For this review, take the finished solid that the model builds, in its own axes (mm). Face numbers are marked on the shaded views. A direction names the side the tool comes from. Give positions to 0.01 mm unless a question says otherwise; leave off trailing zeros. Order: outer loops, then holes, each group sorted by start corner. A loop starts at its lowest first (then second) coordinate and runs counter-clockwise, first axis right, second up. Notation, with made-up numbers: (29.5, 79) - (33.5, 79) arc R23 ccw to (33.5, 101) - close; hole circle Ø5 at (85, 13.5). An arc over 180 degrees is marked (long way). One line per item, written item: value.
Solid Edge part; units mm, degrees
sketch "Sketch1" plane through (0, 0, 0) normal (0, -1, 0) x (1, 0, 0)
  circle A0 centre (0, 0) radius 125
extrude "Protrusion1" add sketch "Sketch1" against normal blind 6
sketch "Sketch2" plane through (0, 0, 0) normal (0, -1, 0) x (1, 0, 0)
  circle A0 centre (0, 0) radius 25
extrude "ProtrusiónExtruida_2" add sketch "Sketch2" along normal blind 45
sketch "Sketch3" plane through (0, -45, 0) normal (0, -1, 0) x (1, 0, 0)
  line L0 (-5, 24.4949) -> (-5, 16.7705)
  line L1 (5, 24.4949) -> (5, 16.7705)
  arc A0 (5, 24.4949) -> (-5, 24.4949) centre (0, 0) cw
  arc A1 (5, 16.7705) -> (-5, 16.7705) centre (0, 0) cw
extrude "Cutout1" cut sketch "Sketch3" against normal up to surface (45 mm away)
sketch "Sketch4" plane through (0, 0, 0) normal (0, -1, 0) x (1, 0, 0)
  circle A0 centre (0, 0) radius 25
extrude "ProtrusiónExtruida_3" add sketch "Sketch4" along normal blind 15
fillet "Redondeo_1" radius 5 1 edges at (-25, 0, 0)
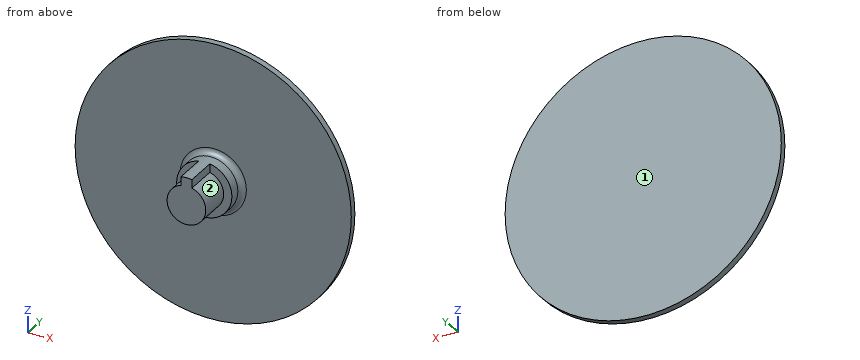
(1) Wall thickness on line 1 (X direction, y = -32, z = -0.5); line 2 (Y direction, x = 111.5, z = 41); line 3 (X direction, y = -10.5, z = 21.5): over which ranges is each line inside the solid? List them lowest first. Write a range as from..to.
Answers below:
line 1: x = -17.49..17.49
line 2: y = 0..6
line 3: x = -12.76..12.76
(2) Take a section at C-C (y = -38). Write out the cut boundary in (x, z).
Answers below:
outline: (-5, 16.77) arc R17.5 ccw (long way) to (5, 16.77) - (5, 24.49) arc R25 ccw to (-5, 24.49) - close
(3) Take a section at D-D (z = -74). Write out the cut boundary in (x, y), then the cut area to 3 significant figures.
Answers below:
outline: (-100.74, 0) - (100.74, 0) - (100.74, 6) - (-100.74, 6) - close
area: 1,210 mm^2
(4) For P1, Ø4, axis at y = -34.5, z = 19.5, coming from the -X side; P2, Ø6, axis at y = -27, z = 20.5, coming from the +X side; P3, Ø12, axis at x = 9.5, y = -17, coming from the -Z side, all flat-tipped, find the tip position at first contact; note any pin that passes through.
Answers below:
P1: stops at x = -5
P2: stops at x = 5
P3: stops at z = -24.7
(5) Take a section at B-B (z = 0). Write out the cut boundary in (x, y).
Answers below:
outline: (-125, 0) - (-30, 0) arc R5 cw to (-25, -5) - (-25, -15) - (-17.5, -15) - (-17.5, -45) - (17.5, -45) - (17.5, -15) - (25, -15) - (25, -5) arc R5 cw to (30, 0) - (125, 0) - (125, 6) - (-125, 6) - close
(6) Take a section at A-A (x = 0). Write out the cut boundary in (y, z).
Answers below:
outline: (-45, -17.5) - (-15, -17.5) - (-15, -25) - (-5, -25) arc R5 cw to (0, -30) - (0, -125) - (6, -125) - (6, 125) - (0, 125) - (0, 30) arc R5 cw to (-5, 25) - (-45, 25) - close
(7) Machinability: for the marked faces 1 and 2, which of the approach directions +Z, -Z, +X, -X, +Y, -Y give a long, thin tool a straight path to every point of the face, cutting with its end or side? Answer none if there is none.
Answers below:
face 1: +Z, -Z, +X, -X, +Y
face 2: -Y
